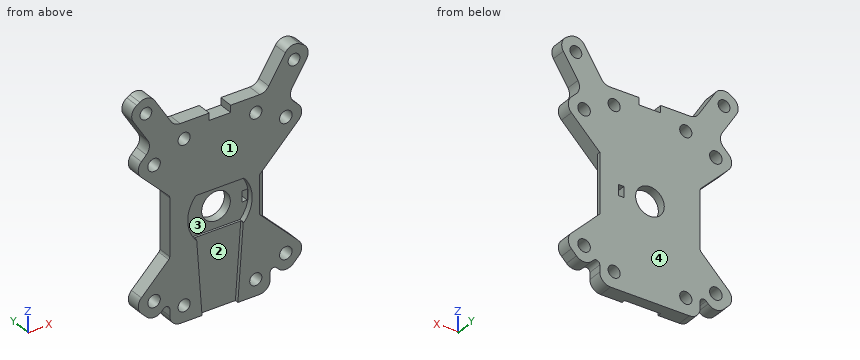
from build123d import *

# Parameters (mm, degrees)
SKETCH1_W           = 28
SKETCH1_H           = 54
BOSS_EXTRUDE1_DEPTH = 4
BOSS_EXTRUDE4_DEPTH = 4
SKETCH2_R           = 1.75
BOSS_EXTRUDE2_DEPTH = 4
SKETCH3_R           = 1.7
CUT_EXTRUDE1_DEPTH  = 4
CUT_EXTRUDE2_REACH  = 48.344
SKETCH4_R           = 4
SKETCH4_W           = 1.5
SKETCH4_H           = 3
CUT_EXTRUDE3_DEPTH  = 1.6
CHAMFER1_SIZE       = 3
FILLET1_R           = 3
FILLET2_R           = 1
SKETCH7_W           = 6
SKETCH7_H           = 4
CUT_EXTRUDE4_DEPTH  = 2
CUT_EXTRUDE5_DEPTH  = 1
CUT_EXTRUDE6_REACH  = 46.778
SKETCH9_R           = 1.65


with BuildPart() as part:
    # Sketch1 → Boss-Extrude1 (new body)
    with BuildSketch(Plane(origin=(0, 0, 0), x_dir=(1, 0, 0), z_dir=(0, 1, 0))):
        Rectangle(SKETCH1_W, SKETCH1_H)
    extrude(amount=BOSS_EXTRUDE1_DEPTH)

    # Sketch10 → Boss-Extrude4 (add)
    with BuildSketch(Plane(origin=(0, 0, 0), x_dir=(1, 0, 0), z_dir=(0, 1, 0))):
        Polygon((2.968168337, 1.854717425), (0, 0), (2.968168337, -1.854717425), (0, -6.604779702), (19.818360025, -38.32078556), (25.754696699, -34.61135071), align=None)
        Polygon((0, -6.604779702), (-2.968168337, -1.854717425), (0, 0), (-2.968168337, 1.854717425), (-25.754696699, -34.61135071), (-19.818360025, -38.32078556), align=None)
    extrude(amount=BOSS_EXTRUDE4_DEPTH)

    # Sketch2 → Boss-Extrude2 (add)
    # profile 1 of 4: a face of its own
    with BuildSketch(Plane(origin=(0, 0, 0), x_dir=(1, 0, 0), z_dir=(0, 1, 0))):
        Polygon((14, 19.656854249), (14, 8.343145751), (24.04163056, 18.384776311), (18.384776311, 24.04163056), align=None)
        with Locations(Location((18.384776311, 18.384776311, 0), (0, 0, 270))):
            Circle(SKETCH2_R, mode=Mode.SUBTRACT)
    # profile 2 of 4: a face of its own
    with BuildSketch(Plane(origin=(0, 0, 0), x_dir=(1, 0, 0), z_dir=(0, 1, 0))):
        Polygon((24.04163056, -18.384776311), (14, -8.343145751), (14, -15.799903705), (18.85572261, -23.570684261), align=None)
        with Locations(Location((18.384776311, -18.384776311, 0), (0, 0, 270))):
            Circle(SKETCH2_R, mode=Mode.SUBTRACT)
    # profile 3 of 4: a face of its own
    with BuildSketch(Plane(origin=(0, 0, 0), x_dir=(1, 0, 0), z_dir=(0, 1, 0))):
        Polygon((-24.04163056, -18.384776311), (-18.85572261, -23.570684261), (-14, -15.799903705), (-14, -8.343145751), align=None)
        with Locations(Location((-18.384776311, -18.384776311, 0), (0, 0, 270))):
            Circle(SKETCH2_R, mode=Mode.SUBTRACT)
    # profile 4 of 4: a face of its own
    with BuildSketch(Plane(origin=(0, 0, 0), x_dir=(1, 0, 0), z_dir=(0, 1, 0))):
        Polygon((-14, 8.343145751), (-14, 19.656854249), (-18.384776311, 24.04163056), (-24.04163056, 18.384776311), align=None)
        with Locations(Location((-18.384776311, 18.384776311, 0), (0, 0, 270))):
            Circle(SKETCH2_R, mode=Mode.SUBTRACT)
    extrude(amount=BOSS_EXTRUDE2_DEPTH)

    # Sketch3 → Cut-Extrude1 (cut)
    with BuildSketch(Plane(origin=(0, 4, 0), x_dir=(1, 0, 0), z_dir=(0, 1, 0))):
        with Locations(Location((10, -22.5, 0), (0, 0, 270))):
            Circle(SKETCH3_R)
        with Locations(Location((-10, -22.5, 0), (0, 0, 270))):
            Circle(SKETCH3_R)
        with Locations(Location((-10, 22.5, 0), (0, 0, 270))):
            Circle(SKETCH3_R)
        with Locations(Location((10, 22.5, 0), (0, 0, 270))):
            Circle(SKETCH3_R)
    extrude(amount=-CUT_EXTRUDE1_DEPTH, mode=Mode.SUBTRACT)

    # Sketch4 → Cut-Extrude2 (cut, up to next)
    with BuildSketch(Plane(origin=(0, 4, 0), x_dir=(1, 0, 0), z_dir=(0, 1, 0)), mode=Mode.PRIVATE) as cut_extrude2_sk1:
        with Locations(Location((0, 0, 0), (0, 0, 270))):
            Circle(SKETCH4_R)
    cut_extrude2_tool1 = extrude(cut_extrude2_sk1.sketch, amount=-CUT_EXTRUDE2_REACH, mode=Mode.PRIVATE) & part.part
    # Sketch4 → Cut-Extrude2 (cut, up to next)
    with BuildSketch(Plane(origin=(0, 4, 0), x_dir=(1, 0, 0), z_dir=(0, 1, 0)), mode=Mode.PRIVATE) as cut_extrude2_sk2:
        with Locations((8, 0)):
            Rectangle(SKETCH4_W, SKETCH4_H)
    cut_extrude2_tool2 = extrude(cut_extrude2_sk2.sketch, amount=-CUT_EXTRUDE2_REACH, mode=Mode.PRIVATE) & part.part
    add(cut_extrude2_tool1.solids().sort_by_distance((0, 4, 0))[0], mode=Mode.SUBTRACT)
    add(cut_extrude2_tool2.solids().sort_by_distance((8, 4, 0))[0], mode=Mode.SUBTRACT)

    # Sketch5 → Cut-Extrude3 (cut)
    with BuildSketch(Plane.XZ):
        with BuildLine():
            Line((6.708203932, -6), (-6.708203932, -6))
            ThreePointArc((-6.708203932, -6), (-9, 0), (-6.708203932, 6))
            Line((-6.708203932, 6), (6.708203932, 6))
            ThreePointArc((6.708203932, 6), (9, 0), (6.708203932, -6))
        make_face()
    extrude(amount=-CUT_EXTRUDE3_DEPTH, mode=Mode.SUBTRACT)

    # Chamfer1
    chamfer1_edges = [part.edges().sort_by_distance(p)[0] for p in [
        (14, 0, 0),
    ]]
    chamfer(chamfer1_edges, length=CHAMFER1_SIZE)

    # Fillet1
    fillet1_edges = [part.edges().sort_by_distance(p)[0] for p in [
        (18.384776311, 2, -24.04163056),
        (24.04163056, 2, -18.384776311),
        (18.85572261, 2, 23.570684261),
        (24.04163056, 2, 18.384776311),
        (-18.85572261, 2, 23.570684261),
        (-24.04163056, 2, 18.384776311),
        (12.74434809, 2, 27),
        (25.754696699, 2, 34.61135071),
        (19.818360025, 2, 38.32078556),
        (-19.818360025, 2, 38.32078556),
        (-25.754696699, 2, 34.61135071),
        (-12.74434809, 2, 27),
        (-14, 2, -27),
        (-24.04163056, 2, -18.384776311),
        (14, 2, -27),
        (-18.384776311, 2, -24.04163056),
    ]]
    fillet(fillet1_edges, radius=FILLET1_R)

    # Fillet2
    fillet2_edges = [part.edges().sort_by_distance(p)[0] for p in [
        (14, 2, -19.656854249),
        (-14, 2, 8.343145751),
        (-14, 2, -19.656854249),
        (-14, 2, -8.343145751),
    ]]
    fillet(fillet2_edges, radius=FILLET2_R)

    # Sketch7 → Cut-Extrude4 (cut)
    with BuildSketch(Plane.XY.offset(27)):
        with Locations((0, 2)):
            Rectangle(SKETCH7_W, SKETCH7_H)
    extrude(amount=-CUT_EXTRUDE4_DEPTH, mode=Mode.SUBTRACT)

    # Sketch8 → Cut-Extrude5 (cut)
    with BuildSketch(Plane(origin=(0, 0, 0), x_dir=(-1, 0, 0), z_dir=(0, 1, 0))):
        Polygon((-5, -27), (5, -27), (6.5, -6), (-6.5, -6), align=None)
    extrude(amount=CUT_EXTRUDE5_DEPTH, mode=Mode.SUBTRACT)

    # Sketch9 → Cut-Extrude6 (cut, up to next)
    with BuildSketch(Plane(origin=(0, 4, 0), x_dir=(1, 0, 0), z_dir=(0, 1, 0)), mode=Mode.PRIVATE) as cut_extrude6_sk1:
        with Locations(Location((20.666851305, -33.07387575, 0), (0, 0, 270))):
            Circle(SKETCH9_R)
    cut_extrude6_tool1 = extrude(cut_extrude6_sk1.sketch, amount=-CUT_EXTRUDE6_REACH, mode=Mode.PRIVATE) & part.part
    # Sketch9 → Cut-Extrude6 (cut, up to next)
    with BuildSketch(Plane(origin=(0, 4, 0), x_dir=(1, 0, 0), z_dir=(0, 1, 0)), mode=Mode.PRIVATE) as cut_extrude6_sk2:
        with Locations(Location((-20.666851305, -33.07387575, 0), (0, 0, 90))):
            Circle(SKETCH9_R)
    cut_extrude6_tool2 = extrude(cut_extrude6_sk2.sketch, amount=-CUT_EXTRUDE6_REACH, mode=Mode.PRIVATE) & part.part
    add(cut_extrude6_tool1.solids().sort_by_distance((20.666851, 4, 33.073876))[0], mode=Mode.SUBTRACT)
    add(cut_extrude6_tool2.solids().sort_by_distance((-20.666851, 4, 33.073876))[0], mode=Mode.SUBTRACT)


solid = part.part
The listing builds one solid part. Answer for the finished solid, in the listing's coordinates (mm). Face numbers are marked on the shaded views. A direction names the side the tool comes from. Give positions to 0.01 mm unless a question says otherwise; leave off trailing zeros. Write each loop counter-clockwise with the first axis right and the second up, starting at its lowest first coordinate (ties: lowest second). Pieces come first, ordered by that corner, then holes.
Item 1: Find the intervals of material crossed by line 1 along X through (y, z) = (0.35, -21.5); line 2 along Z through (x, y) = (18.5, 0.2); line 3 along X through (y, z) = (3.15, 22), in increasing order.
Item 2: Section D-D, the plane y = 2.35 is taken. Count the separate pieces of the cut face and the enclosed holes in it, plus the area to 3 significant figures.
Item 3: Flat-ended cylindrical pins translate along their axes: P1, Ø6, axis at x = 2.5, z = 0.5, coming from the -Y side; P2, Ø0.7, axis at y = 3, z = 0, coming from the -X side; P3, Ø2, axis at y = 2, z = 29.5, coming from the +X side. Find the tip coordinate at first contact, or state that the pin passes through.
Item 4: Determine the mould class of the marked faces 3 and 4 for opening direction Z: released by +Z, released by -Z, zero draft, split by the parting line, or undercut.
Item 5: Which of the six approach directions +Z, -Z, +X, -X, +Y, -Y give full straight-line access (tool end or side, diameter ignored) to the marked faces 1 and 2?
Item 6: Section C-C, the plane x = -10 is taken. Write down the section's boundary in (y, z).
Item 7: Section B-B, the plane x = 0 is taken. Write down the section's boundary in (y, z), plus the area to 3 significant figures.
Item 8: Section A-A, the plane z = 0 is taken. Write down the section's boundary in (x, y).
Completed:
1. line 1: x = -20.93 to -15.84, -14.18 to -11.37, -8.63 to -5.39, 5.39 to 8.63, 11.37 to 14.18, 15.84 to 20.93
1. line 2: z = -22.8 to -20.13, -16.64 to -12.84, 12.84 to 16.64, 20.13 to 36.15
1. line 3: x = -20.43 to -11.62, -8.38 to 8.38, 11.62 to 20.43
2. separate pieces: 1
2. enclosed holes: 12
2. area: 1,860 mm2
3. P1: stops at y = 1.6
3. P2: stops at x = -14
3. P3: stops at x = 23.19
4. face 3: undercut
4. face 4: zero draft
5. face 1: +Z, -Z, +X, -X, -Y
5. face 2: -Y
6. outline: (0, -27) - (4, -27) - (4, -24.2) - (0, -24.2) - close; (0, -20.8) - (4, -20.8) - (4, 20.8) - (0, 20.8) - close; (0, 24.2) - (4, 24.2) - (4, 27) - (0, 27) - close
7. outline: (0, 6) - (1.6, 6) - (1.6, 4) - (4, 4) - (4, 25) - (0, 25) - close; (1, -27) - (4, -27) - (4, -4) - (1.6, -4) - (1.6, -6) - (1, -6) - close
7. area: 149 mm2
8. outline: (-14, 0) - (-9, 0) - (-9, 1.6) - (-4, 1.6) - (-4, 4) - (-14, 4) - close; (4, 1.6) - (7.25, 1.6) - (7.25, 4) - (4, 4) - close; (8.75, 1.6) - (9, 1.6) - (9, 0) - (11, 0) - (14, 3) - (14, 4) - (8.75, 4) - close
